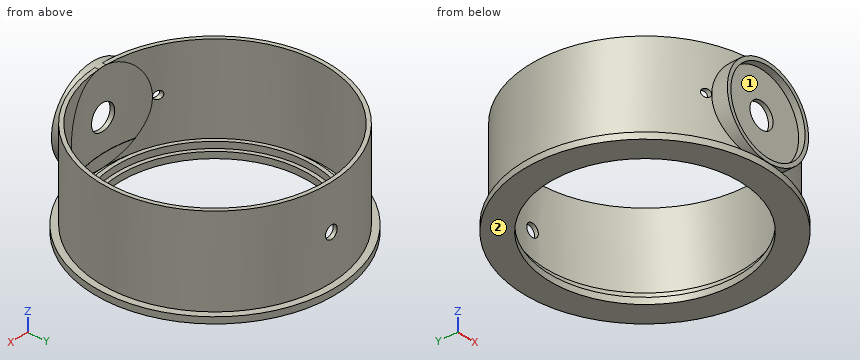
```python
from build123d import *

# Parameters (mm, degrees)
SKETCH2_R           = 95
SKETCH2_R_2         = 75
BOSS_EXTRUDE1_DEPTH = 5
SKETCH3_R           = 90
SKETCH3_R_2         = 87
BOSS_EXTRUDE2_DEPTH = 75
SKETCH4_R           = 81
SKETCH4_R_2         = 78
BOSS_EXTRUDE4_DEPTH = 10
SKETCH6_R           = 35
BOSS_EXTRUDE5_DEPTH = 95
SKETCH7_R           = 75
CUT_EXTRUDE1_DEPTH  = 95
SKETCH8_R           = 87
CUT_EXTRUDE3_DEPTH  = 95
SKETCH9_R           = 86.82735855
CUT_EXTRUDE4_DEPTH  = 10
SKETCH10_R          = 81
SKETCH10_R_2        = 78
BOSS_EXTRUDE6_DEPTH = 10
SKETCH11_R          = 32
CUT_EXTRUDE5_DEPTH  = 5
SKETCH12_R          = 10
CUT_EXTRUDE6_DEPTH  = 5
SKETCH13_R          = 5
CUT_EXTRUDE7_DEPTH  = 185
SKETCH14_R          = 3.11609281
CUT_EXTRUDE9_DEPTH  = 185


with BuildPart() as part:
    # Sketch2 → Boss-Extrude1 (new body)
    with BuildSketch(Plane.XY):
        Circle(SKETCH2_R)
        Circle(SKETCH2_R_2, mode=Mode.SUBTRACT)
    extrude(amount=BOSS_EXTRUDE1_DEPTH)

    # Sketch3 → Boss-Extrude2 (add)
    with BuildSketch(Plane.XY):
        Circle(SKETCH3_R)
        Circle(SKETCH3_R_2, mode=Mode.SUBTRACT)
    extrude(amount=BOSS_EXTRUDE2_DEPTH)

    # Sketch4 → Boss-Extrude4 (add)
    with BuildSketch(Plane.XY):
        Circle(SKETCH4_R)
        Circle(SKETCH4_R_2, mode=Mode.SUBTRACT)
    extrude(amount=BOSS_EXTRUDE4_DEPTH)

    # Sketch6 → Boss-Extrude5 (add)
    with BuildSketch(Plane(origin=(0, 0, 0), x_dir=(1, 0, 0), z_dir=(0, 1, 0))):
        with Locations(Location((0, -40.143816704, 0), (0, 0, 270))):
            Circle(SKETCH6_R)
    extrude(amount=-BOSS_EXTRUDE5_DEPTH)

    # Sketch7 → Cut-Extrude1 (cut)
    with BuildSketch(Plane.XY):
        Circle(SKETCH7_R)
    extrude(amount=CUT_EXTRUDE1_DEPTH, mode=Mode.SUBTRACT)

    # Sketch8 → Cut-Extrude3 (cut)
    with BuildSketch(Plane.XY.offset(15)):
        with Locations(Location((0, 0, 0), (0, 0, 267.912115018))):
            Circle(SKETCH8_R)
    extrude(amount=CUT_EXTRUDE3_DEPTH, mode=Mode.SUBTRACT)

    # Sketch9 → Cut-Extrude4 (cut)
    with BuildSketch(Plane.XY.offset(15)):
        Circle(SKETCH9_R)
    extrude(amount=-CUT_EXTRUDE4_DEPTH, mode=Mode.SUBTRACT)

    # Sketch10 → Boss-Extrude6 (add)
    with BuildSketch(Plane.XY):
        Circle(SKETCH10_R)
        Circle(SKETCH10_R_2, mode=Mode.SUBTRACT)
    extrude(amount=BOSS_EXTRUDE6_DEPTH)

    # Sketch11 → Cut-Extrude5 (cut)
    with BuildSketch(Plane.XZ.offset(95)):
        with Locations(Location((0, 40.143816704, 0), (0, 0, 270))):
            Circle(SKETCH11_R)
    extrude(amount=-CUT_EXTRUDE5_DEPTH, mode=Mode.SUBTRACT)

    # Sketch12 → Cut-Extrude6 (cut)
    with BuildSketch(Plane.XZ.offset(90)):
        with Locations(Location((0, 40.143816704, 0), (0, 0, 270))):
            Circle(SKETCH12_R)
    extrude(amount=-CUT_EXTRUDE6_DEPTH, mode=Mode.SUBTRACT)

    # Sketch13 → Cut-Extrude7 (cut)
    with BuildSketch(Plane.XZ.offset(90)):
        with Locations(Location((0, 40.143816704, 0), (0, 0, 270))):
            Circle(SKETCH13_R)
    extrude(amount=-CUT_EXTRUDE7_DEPTH, mode=Mode.SUBTRACT)

    # Sketch14 → Cut-Extrude9 (cut)
    with BuildSketch(Plane(origin=(0, 0, 0), x_dir=(1, 0, 0), z_dir=(0, 1, 0))):
        with Locations(Location((-38.2, -40.29848956, 0), (0, 0, 270))):
            Circle(SKETCH14_R)
    extrude(amount=-CUT_EXTRUDE9_DEPTH, mode=Mode.SUBTRACT)


solid = part.part
```
Geometry check sheet. Reference: the model listing, model coordinates, mm. Face numbers are marked on the shaded views. A direction names the side the tool comes from. Round coordinates to 2 decimals unless told otherwise and drop trailing zeros. Order: outer loops, then holes, each group sorted by start corner. A loop starts at its lowest first (then second) coordinate and runs counter-clockwise, first axis right, second up. Notation, with made-up numbers: (-19.75, -1.75) - (-1.75, -1.75) arc R28 ccw to (-1.75, 20.25) - close; hole circle Ø3 at (-25, 77.25). An arc over 180 degrees is marked (long way). Use a Markdown table: item, result. Add a question column.
(1) Sectioned sample at D-D, the plane z = 27. Enter the section's corners in (x, y), and give its area (3 significant figures).
(2) Sectioned sample at A-A, the plane y = 0. Enter the section's corners in (x, z).
(3) Sectioned sample at B-B, the plane z = 40. Enter the section's corners in (x, y), and give its area (3 significant figures).
(4) Tool access check on the marked faces 1 and 2. Record the directions out of +Z, -Z, +X, -X, +Y, -Y that give a thin tool (end or side, any length) a straight path to the whole face; none if there is none.
(5) Depth check by flat-ended pin: pin 1 (2 mm diameter, centred on y = -61.5, z = 14.5, fed in from -X); pin 2 (1.8 mm diameter, centred on x = -9.5, y = -85, fed in from +Z); pin 3 (6 mm diameter, centred on y = 71, z = 67, fed in from +X). Enter the tip coordinate at first touch or a pass-through.
(6) Material ranges on line 1 along Y through (x, z) = (0, 6.65); line 2 along X through (y, z) = (0, 8.7); line 3 along Z through (x, y) = (0, 89.35), recorded low to high. Write a range as [from, to].
(7) Sectioned sample at C-C, the plane x = -38.2. Enter the section's corners in (y, z), and give its area (3 significant figures).
Answers below:
| question | item | result |
|---|---|---|
| 1 | outline | (-32.44, -95) - (-29.18, -95) - (-29.18, -90) - (29.18, -90) - (29.18, -95) - (32.44, -95) - (32.44, -83.95) arc R90 ccw (long way) to (-32.44, -83.95) - close; hole circle Ø174 at (0, 0) |
| 1 | area | 1,830 mm² |
| 2 | outline | (-95, 0) - (-75, 0) - (-75, 5) - (-78, 5) - (-78, 10) - (-81, 10) - (-81, 5) - (-87, 5) - (-87, 75) - (-90, 75) - (-90, 5) - (-95, 5) - close; (75, 0) - (95, 0) - (95, 5) - (90, 5) - (90, 75) - (87, 75) - (87, 5) - (81, 5) - (81, 10) - (78, 10) - (78, 5) - (75, 5) - close |
| 3 | outline | (-41.3, -79.96) - (-41.3, -76.57) arc R87 cw to (-5, 86.86) - (-5, 89.86) arc R90 ccw to start; (-35.1, -82.87) arc R90 ccw to (-35, -82.92) - (-35, -95) - (-32, -95) - (-32, -90) - (-10, -90) - (-10, -86.42) arc R87 cw to (-35.1, -79.61) - close; (5, 86.86) arc R87 cw to (10, -86.42) - (10, -90) - (32, -90) - (32, -95) - (35, -95) - (35, -82.92) arc R90 ccw to (5, 89.86) - close |
| 3 | area | 1,750 mm² |
| 4 | face 1 | -Y |
| 4 | face 2 | -Z, +X, -X, +Y, -Y |
| 5 | pin 1 | x = -66.63 |
| 5 | pin 2 | z = 5 |
| 5 | pin 3 | x = 58.96 |
| 6 | line 1 | [-95, -86.83], [-81, -78], [78, 81], [87, 90] |
| 6 | line 2 | [-90, -87], [-81, -78], [78, 81], [87, 90] |
| 6 | line 3 | [0, 35.14], [45.14, 75] |
| 7 | outline | (-86.98, 0) - (-64.54, 0) - (-64.54, 5) - (-68.01, 5) - (-68.01, 10) - (-71.43, 10) - (-71.43, 5) - (-78.16, 5) - (-78.16, 37.18) - (-81.49, 37.18) - (-81.49, 5) - (-86.98, 5) - close; (-81.49, 43.41) - (-78.16, 43.41) - (-78.16, 75) - (-81.49, 75) - close; (64.54, 0) - (86.98, 0) - (86.98, 5) - (81.49, 5) - (81.49, 75) - (78.16, 75) - (78.16, 5) - (71.43, 5) - (71.43, 10) - (68.01, 10) - (68.01, 5) - (64.54, 5) - close |
| 7 | area | 703 mm² |
